Build history of the part. All positions in model axes, mm. A direction names the side the tool comes from. Coordinates: 2 decimals unless noted, no trailing zeros. Order: outer loops, then holes, each group sorted by start corner. A loop starts at its lowest first (then second) coordinate and runs counter-clockwise, first axis right, second up. Notation, with made-up numbers: (-11.5, 63.25) - (39.5, 63.25) arc R13 cw to (39.5, 81.25) - close; hole circle Ø10 at (-23.75, -20). An arc over 180 degrees is marked (long way). One line per item, written item: value.
from build123d import *

# Parameters (mm, degrees)
SKETCH_W     = 47
SKETCH_H     = 40
SKETCH_R     = 2
PAD_DEPTH    = 2
PAD001_DEPTH = 15
SKETCH002_W  = 4.5
SKETCH002_H  = 20
PAD002_DEPTH = 2


with BuildPart() as part:
    # Sketch → Pad (new body)
    with BuildSketch(Plane.XY):
        Rectangle(SKETCH_W, SKETCH_H)
        with Locations((-18.485281, -14.985281)):
            Circle(SKETCH_R, mode=Mode.SUBTRACT)
        with Locations((18.485281, -14.985281)):
            Circle(SKETCH_R, mode=Mode.SUBTRACT)
    extrude(amount=PAD_DEPTH)

    # Sketch001 (on Face8 of Pad) → Pad001 (join)
    with BuildSketch(Plane.XY.offset(2)):
        Polygon((-23.5, -20), (23.5, -20), (23.5, 20), (22, 20), (22, -18.5), (-22, -18.5), (-22, 20), (-23.5, 20), align=None)
    extrude(amount=PAD001_DEPTH)

    # Sketch002 (on Face14 of Pad001) → Pad002 (join)
    with BuildSketch(Plane.XY.offset(17)):
        with Locations((-21.25, 10)):
            Rectangle(SKETCH002_W, SKETCH002_H)
        with Locations((21.25, 10)):
            Rectangle(SKETCH002_W, SKETCH002_H)
    extrude(amount=PAD002_DEPTH)


solid = part.part
1. Band-saw the part on B-B, the plane x = 18. Give the cut face in (y, z), and give its area (3 significant figures).
Values found:
outline: (-20, 0) - (-16.93, 0) - (-16.93, 2) - (-18.5, 2) - (-18.5, 17) - (-20, 17) - close; (-13.05, 0) - (20, 0) - (20, 2) - (-13.05, 2) - close
area: 94.7 mm2
2. Two-plate mould, pull along X, no slides. Class faces 1 (the face through (0, -18.5, 9)), 2 (the face through (-23.5, 0, 9)), 3 (the face through (23.5, 0, 9)), 4 (the face through (21, 10, 19)): pulls with the +X half, pulls with the -X half, needs draft (parallel to the pull), parting line crosses it, or undercut.
Values found:
face 1: undercut
face 2: pulls with the -X half
face 3: pulls with the +X half
face 4: needs draft
3. Band-saw the part on C-C, the plane y = -10. Give the cut face in (x, z).
Values found:
outline: (-23.5, 0) - (23.5, 0) - (23.5, 17) - (22, 17) - (22, 2) - (-22, 2) - (-22, 17) - (-23.5, 17) - close
4. 3-axis set-ups, long thin cutter, end or side, ignore diameter. For faces 5 (the face through (0, 0, 0)), 6 (the face through (19, 10, 18)), 7 (the face through (21, 0, 18)), 8 (the face through (20, 10, 17)): which of +Z, -Z, +X, -X, +Y, -Y reach the whole face in a straight line?
Values found:
face 5: -Z, +X, -X, +Y, -Y
face 6: +Z, +Y, -Y
face 7: +Z, +X, -X, -Y
face 8: +Y
5. Band-saw the part on A-A, the plane z = 15.25. Give the cut face in (x, y).
Values found:
outline: (-23.5, -20) - (23.5, -20) - (23.5, 20) - (22, 20) - (22, -18.5) - (-22, -18.5) - (-22, 20) - (-23.5, 20) - close
6. Band-saw the part on D-D, the plane x = -12.5. Give the cut face in (y, z).
Values found:
outline: (-20, 0) - (20, 0) - (20, 2) - (-18.5, 2) - (-18.5, 17) - (-20, 17) - close
7. Flat gauge pins, fed straight in: P1, Ø1.6, axis at x = 20.5, z = 18.5, coming from the -Y side; P2, Ø16, axis at x = -4.5, y = -14, coming from the +Z side; P3, Ø1.5, axis at x = -8, z = 13.5, coming from the +Y side. Where does each tip first touch, or does it go through?
Values found:
P1: stops at y = 0
P2: stops at z = 17
P3: stops at y = -18.5
8. Probe line 1 along X through (y, z) = (17, 15.5); line 2 along Y through (x, z) = (-10, 9.25); line 3 along Z through (x, y) = (-13.5, -16.5). List the from-to ranges inside material, lowest first.
Values found:
line 1: x = -23.5 to -22, 22 to 23.5
line 2: y = -20 to -18.5
line 3: z = 0 to 2
